from build123d import *


with BuildPart() as part:
    # BodySke → BaseBody (revolve)
    with BuildSketch(Plane.XY, mode=Mode.PRIVATE) as basebody_sk:
        with BuildLine():
            Line((17, 8.633974596), (14.633974596, 10))
            Line((14.633974596, 10), (1.5, 10))
            Line((1.5, 10), (0, 8.5))
            Line((0, 8.5), (0, 0))
            Line((0, 0), (120, 0))
            Line((120, 0), (120, 8.5))
            Line((120, 8.5), (118.5, 10))
            Line((118.5, 10), (97.6, 10))
            Line((97.6, 10), (95.233974596, 8.633974596))
            ThreePointArc((95.233974596, 8.633974596), (94.992793641, 8.534074174), (94.733974596, 8.5))
            Line((94.733974596, 8.5), (93.501923789, 8.5))
            ThreePointArc((93.501923789, 8.5), (92.794817007, 8.792893219), (92.501923789, 9.5))
            Line((92.501923789, 9.5), (92.501923789, 10))
            Line((92.501923789, 10), (20, 10))
            Line((20, 10), (20, 9.5))
            ThreePointArc((20, 9.5), (19.707106781, 8.792893219), (19, 8.5))
            Line((19, 8.5), (17.5, 8.5))
            ThreePointArc((17.5, 8.5), (17.241180955, 8.534074174), (17, 8.633974596))
        make_face()
    revolve(basebody_sk.sketch.rotate(Axis((-3.175, 0, 0), (1, 0, 0)), 90), axis=Axis((-3.175, 0, 0), (1, 0, 0)))


solid = part.part
Design review of the part built by this model. Coordinates are the model's own, in mm. A direction names the side the tool comes from. Round coordinates to 2 decimals unless told otherwise and drop trailing zeros. Order: outer loops, then holes, each group sorted by start corner. A loop starts at its lowest first (then second) coordinate and runs counter-clockwise, first axis right, second up. Notation, with made-up numbers: M -16.5,34.25 L 38.5,34.25 A24 ccw 38.5,66.25 Z; hole C 24.5,5.25 d4. An arc over 180 degrees is marked long. Answer as CSV lines item,"result". Start each with the question number.
1) Wall thickness on line 1 along X through (y, z) = (-7, 7); line 2 along X through (y, z) = (8.5, 3); line 3 along Y through (x, z) = (30, -2.5): over which ranges is each line inside the solid? List them lowest first. Write a range as [from, to].
2) The part is to be moulded in two halves that separate along X. For faces 1 (the face through (108, 0, -10)), 2 (the face through (120, 0, 0)), 3 (the face through (94.109, -8.428, -1.107)), say which applies: +X half, -X half, draft (parallel to the pull), parting line (faces both ways), or undercut.
3) For pin 1 Ø4 at (x, y) = (90.5, 5.5) entering from +Z; pin 2 Ø1 at (x, z) = (42, -4) entering from +Y; pin 3 Ø1 at (x, z) = (70.5, -3) entering from -Y, all flat-tipped, find the tip position at first contact; note any pin that passes through.
4) Add section A-A (x = 61.5). Give the boundary of the cut face in (y, z).
5) Tool access review of faces 4 (the face through (18.24, -8.428, -1.107)), 5 (the face through (8, 0, -10)): name each direction out of +Z, -Z, +X, -X, +Y, -Y from which nothing blocks a thin tool from reaching the whole face with its end or side.
Resolved:
1,line 1,"[1.4, 14.81], [20, 92.5], [97.43, 118.6]"
1,line 2,"[0.51, 16.34], [19.87, 92.63], [95.89, 119.49]"
1,line 3,"[-9.68, 9.68]"
2,face 1,"draft"
2,face 2,"+X half"
2,face 3,"undercut"
3,pin 1,"z = 9.37"
3,pin 2,"y = 9.37"
3,pin 3,"y = -9.68"
4,outline,"C 0,0 d20"
5,face 4,"none"
5,face 5,"+X, -X"
